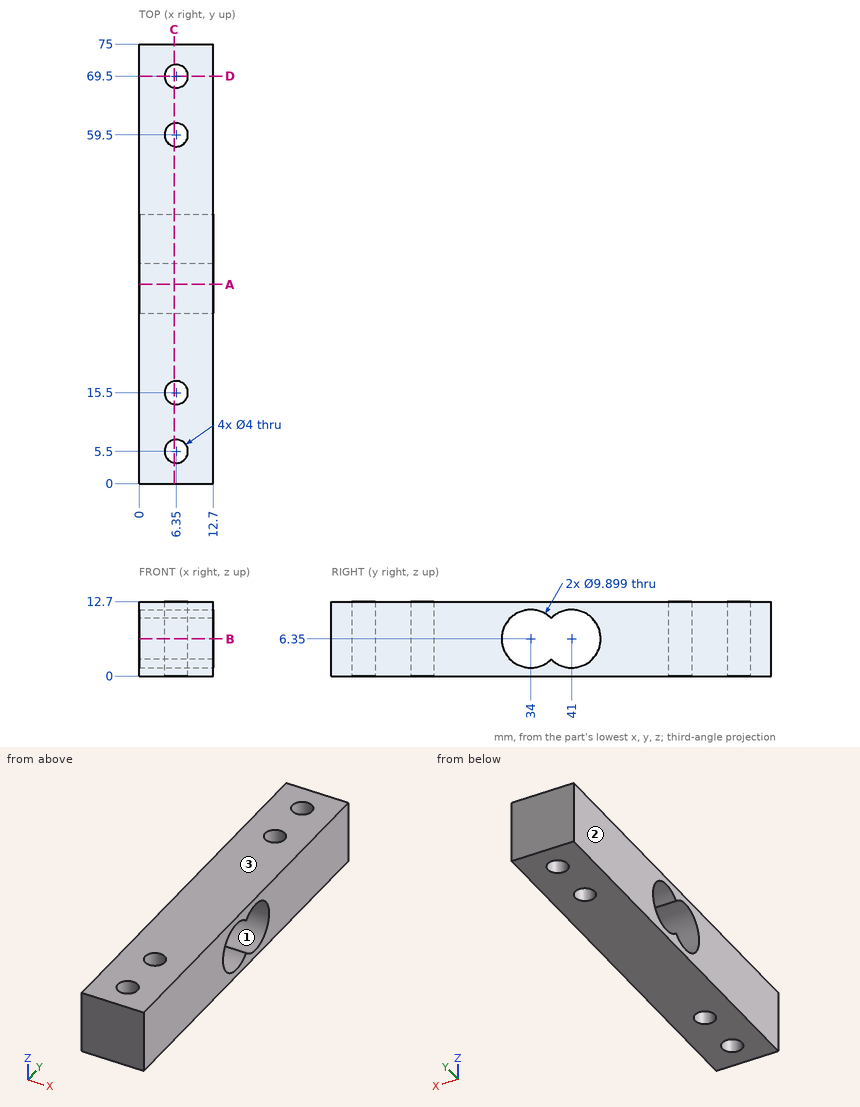
Can you work these out from the drawing? Everything is in mm from the part's minimum corner. Coordinates: 2 decimals unless noted, no trailing zeros. Loops run counter-clockwise (first coordinate to the right, second up) from the corner with the lowest first, then second, coordinate; pieces in that order, holes last.
1. Imagine slicing it at D-D, the plane y = 69.5. Please give me the cut outline in (x, z).
2. Imagine slicing it at C-C, the plane x = 6. Please give me the cut outline in (y, z).
3. If we mould it in two halves opening along Z, with no side actions, what happens to the marked faces 1, 2 and 3? For each: pulls with the +Z half, pulls with the -Z half, needs draft (parallel to the pull), parting line crosses it, or undercut.
4. Imagine slicing it at A-A, the plane y = 34. Please give me the cut outline in (x, z).
5. Imagine slicing it at B-B, the plane z = 6.35. Please give me the cut outline in (x, y).
6. I need wall thicknesses on L1, parallel to Y at x = 8.75, z = 6.5; L2, parallel to Y at x = 2.25, z = 10.5 (1 decimal); L3, parallel to Y at x = 6.35, z = 8.75. Which ranges of each line are inside material? Lowest first, please.
Taken from the geometry:
1. outline: (0, 0) - (4.35, 0) - (4.35, 12.7) - (0, 12.7) - close; (8.35, 0) - (12.7, 0) - (12.7, 12.7) - (8.35, 12.7) - close
2. outline: (0, 0) - (3.53, 0) - (3.53, 12.7) - (0, 12.7) - close; (7.47, 0) - (13.53, 0) - (13.53, 12.7) - (7.47, 12.7) - close; (17.47, 0) - (57.53, 0) - (57.53, 12.7) - (17.47, 12.7) - close; (61.47, 0) - (67.53, 0) - (67.53, 12.7) - (61.47, 12.7) - close; (71.47, 0) - (75, 0) - (75, 12.7) - (71.47, 12.7) - close; hole (37.5, 2.85) arc R4.95 ccw (long way) to (37.5, 9.85) arc R4.95 ccw (long way) to start
3. face 1: undercut
3. face 2: needs draft
3. face 3: pulls with the +Z half
4. outline: (0, 0) - (12.7, 0) - (12.7, 1.4) - (0, 1.4) - close; (0, 11.3) - (12.7, 11.3) - (12.7, 12.7) - (0, 12.7) - close
5. outline: (0, 0) - (12.7, 0) - (12.7, 29.05) - (0, 29.05) - close; (0, 45.95) - (12.7, 45.95) - (12.7, 75) - (0, 75) - close; hole circle Ø4 at (6.35, 5.5); hole circle Ø4 at (6.35, 15.5); hole circle Ø4 at (6.35, 59.5); hole circle Ø4 at (6.35, 69.5)
6. L1: y = 0 to 29.05, 45.95 to 75
6. L2: y = 0 to 31.3, 36.7 to 38.3, 43.7 to 75
6. L3: y = 0 to 3.5, 7.5 to 13.5, 17.5 to 29.67, 45.33 to 57.5, 61.5 to 67.5, 71.5 to 75
